Model file for the job. Use its own axes, mm. Round coordinates to 2 decimals unless told otherwise and drop trailing zeros. Order: outer loops, then holes, each group sorted by start corner. A loop starts at its lowest first (then second) coordinate and runs counter-clockwise, first axis right, second up. Notation, with made-up numbers: (2, 15) - (24, 15) arc R19 cw to (24, 48) - close; hole circle Ø10 at (77.25, 83.25). An arc over 180 degrees is marked (long way). Write item = value, one per line.
```python
from build123d import *

# Parameters (mm, degrees)
F0_R     = 2.413
F0_R_2   = 13.97
F0_R_3   = 14.2875
F1_DEPTH = 6.35
F2_R     = 5.08


# Not quite as in the source:
# - a length typed as a fraction of an inch, garbled in the dataset ("3 / 203.2 mm" for 3/8 in), is restored


with BuildPart() as f1:
    # F0 (on Top) → F1 (new body)
    with BuildSketch(Plane.XY):
        with BuildLine():
            Line((441.7738245296, 37.0731139821), (29.1392452401, 37.0731139821))
            Line((29.1392452401, 37.0731139821), (-39.5561754704, -26.5958569453))
            Line((-39.5561754704, -26.5958569453), (-39.5561754704, -247.4068860179))
            Line((-39.5561754704, -247.4068860179), (21.4038245296, -247.4068860179))
            Line((21.4038245296, -247.4068860179), (21.4038245296, -140.7268860179))
            Line((21.4038245296, -140.7268860179), (222.0638245296, -140.7268860179))
            Line((222.0638245296, -140.7268860179), (222.0638245296, -247.4068860179))
            Line((222.0638245296, -247.4068860179), (333.8238245296, -247.4068860179))
            Line((333.8238245296, -247.4068860179), (333.8238245296, -213.1168860179))
            Line((333.8238245296, -213.1168860179), (359.2238245296, -213.1168860179))
            Line((359.2238245296, -213.1168860179), (359.2238245296, -247.4068860179))
            Line((359.2238245296, -247.4068860179), (448.1238245296, -247.4068860179))
            Line((448.1238245296, -247.4068860179), (448.1238245296, 30.7231139821))
            ThreePointArc((448.1238245296, 30.7231139821), (446.2639525902, 35.2132420426), (441.7738245296, 37.0731139821))
        make_face()
        with Locations((-9.6586965698, -38.8212736462)):
            Circle(F0_R, mode=Mode.SUBTRACT)
        with Locations((26.2623279145, -38.8212736462)):
            Circle(F0_R, mode=Mode.SUBTRACT)
        with Locations((8.3018156723, -20.860761404)):
            Circle(F0_R_2, mode=Mode.SUBTRACT)
        with Locations((-9.6586965698, -2.9002491619)):
            Circle(F0_R, mode=Mode.SUBTRACT)
        with Locations((26.2623279145, -2.9002491619)):
            Circle(F0_R, mode=Mode.SUBTRACT)
        with Locations((102.5335357666, 8.5151046671)):
            Circle(F0_R_3, mode=Mode.SUBTRACT)
        with Locations((320.4351010724, -6.8675098969)):
            Circle(F0_R, mode=Mode.SUBTRACT)
        with Locations((320.4351010724, 26.3149594916)):
            Circle(F0_R, mode=Mode.SUBTRACT)
        with Locations((353.6175704608, -6.8675098969)):
            Circle(F0_R, mode=Mode.SUBTRACT)
        with Locations((337.0263357666, 9.7237247974)):
            Circle(F0_R_2, mode=Mode.SUBTRACT)
        with Locations((353.6175704608, 26.3149594916)):
            Circle(F0_R, mode=Mode.SUBTRACT)
        with Locations((432.7335357666, 4.0531139821)):
            Circle(F0_R_3, mode=Mode.SUBTRACT)
    extrude(amount=F1_DEPTH)

    # F2
    f2_edges = [f1.edges().sort_by_distance(p)[0] for p in [
        (21.403825, -140.726886, 3.175),
        (222.063825, -140.726886, 3.175),
        (333.823825, -213.116886, 3.175),
        (359.223825, -213.116886, 3.175),
    ]]
    fillet(f2_edges, radius=F2_R)


solid = f1.part
```
1) Mould opens along Y. For faces 1 (the face through (446.361, 8.345, 3.131)), 2 (the face through (-4.73, 5.68, 3.13)), 3 (the face through (201, -103, 6.35)) say: +Y half, -Y half, draft (parallel to the pull), parting line (faces both ways), or undercut.
Conclusion:
face_1 = undercut
face_2 = +Y half
face_3 = draft
2) Cut at B-B (z = 4.75). Give the number of separate pieces and of enclosed holes in the cut face, and give its area (3 significant figures).
Conclusion:
separate_pieces = 1
enclosed_holes = 12
area = 112,000 mm^2
3) Cut at C-C (x = 141.5). Write the cut outline in (y, z).
Conclusion:
outline = (-140.73, 0) - (37.07, 0) - (37.07, 6.35) - (-140.73, 6.35) - close
4) Wall check: line 1 along X through (y, z) = (24.5, 3.5); line 2 along X through (y, z) = (-172, 0.5); line 3 along Y through (x, z) = (200.5, 5.5). Give the ranges that are in metal, low to high.
Conclusion:
line_1 = 15.57 to 318.84, 322.03 to 352.03, 355.21 to 448.12
line_2 = -39.56 to 21.4, 222.06 to 448.12
line_3 = -140.73 to 37.07
5) Cut at A-A (y = -227). Write the cut outline in (x, z), and give its area (3 significant figures).
Conclusion:
outline = (-39.56, 0) - (21.4, 0) - (21.4, 6.35) - (-39.56, 6.35) - close; (222.06, 0) - (333.82, 0) - (333.82, 6.35) - (222.06, 6.35) - close; (359.22, 0) - (448.12, 0) - (448.12, 6.35) - (359.22, 6.35) - close
area = 1,660 mm^2
6) Flat gauge pins, fed straight in: pin 1 Ø2 at (y, z) = (4, 3) entering from -X; pin 2 Ø1.5 at (y, z) = (4.5, 1) entering from -X. Where does each tip first touch, or does it go through?
Conclusion:
pin_1 = -7.62
pin_2 = -6.81
